The listing builds one solid part. Answer for the finished solid, in the listing's coordinates (mm). A direction names the side the tool comes from. Coordinates: 2 decimals unless noted, no trailing zeros. Loops run counter-clockwise (first coordinate to the right, second up) from the corner with the lowest first, then second, coordinate; pieces in that order, holes last. Notation, with made-up numbers: M -23.5,6 L 35.5,6 A20 cw 35.5,31 Z; hole C 33,-27.5 d6. An arc over 180 degrees is marked long. Answer in a Markdown table with one row per item. Add a question column.
from build123d import *

# Parameters (mm, degrees)
SKETCH1_R           = 5
BASEHEAD_DEPTH      = 6
SKETCH2_R           = 3
BASEBODY_DEPTH      = 20
HEXAGONSOCKET_DEPTH = 3
TOPFILLET_R         = 0.2
CHAMFER1_SIZE       = 0.1


with BuildPart() as part:
    # Sketch1 → BaseHead (new body)
    with BuildSketch(Plane(origin=(0, 0, 0), x_dir=(0, 0, -1), z_dir=(1, 0, 0))):
        Circle(SKETCH1_R)
    extrude(amount=BASEHEAD_DEPTH)

    # Sketch2 → BaseBody (add)
    with BuildSketch(Plane(origin=(6, 0, 0), x_dir=(0, 0, -1), z_dir=(1, 0, 0))):
        Circle(SKETCH2_R)
    extrude(amount=BASEBODY_DEPTH)

    # Sketch3 → HexagonSocket (cut)
    with BuildSketch(Plane(origin=(0, 0, 0), x_dir=(0, 0, -1), z_dir=(1, 0, 0))):
        Polygon((2.886751346, 0), (1.443375673, 2.5), (-1.443375673, 2.5), (-2.886751346, 0), (-1.443375673, -2.5), (1.443375673, -2.5), align=None)
    extrude(amount=HEXAGONSOCKET_DEPTH, mode=Mode.SUBTRACT)

    # Sketch4 → Cut-Revolve1 (revolve, cut)
    with BuildSketch(Plane(origin=(-4.19613823, 0.75, 0), x_dir=(-1, 0, 0), z_dir=(0, 0, 1))):
        Polygon((-7.19613823, 3.25), (-8.639513903, 0.75), (-7.19613823, 0.75), align=None)
    revolve(axis=Axis((0.838992387, 0, 0), (-1, 0, 0)), mode=Mode.SUBTRACT)

    # TopFillet
    topfillet_edges = [part.edges().sort_by_distance(p)[0] for p in [
        (0, 0, 5),
    ]]
    fillet(topfillet_edges, radius=TOPFILLET_R)

    # Chamfer1
    chamfer1_edges = [part.edges().sort_by_distance(p)[0] for p in [
        (26, 0, 3),
    ]]
    chamfer(chamfer1_edges, length=CHAMFER1_SIZE)


solid = part.part
(1) A cutting plane is placed at A-A (x = 2.25). Give the vertices of the cut face in (y, z).
(2) A cutting plane is placed at C-C (x = 5.5). Give the vertices of the cut face in (y, z), plus the area to 3 significant figures.
(3) For faces 1 (the face through (3.06, -4.88, 1.08)), 2 (the face through (6, -3.3, 0.1)), 3 (the face through (1.479, 1.233, -2.175)), determine the directions among +Z, -Z, +X, -X, +Y, -Y from which every point of the face is accessible in a straight line to the end or side of a thin tool.
(4) A cutting plane is placed at B-B (x = 18). Give the vertices of the cut face in (y, z), plus the area to 3 significant figures.
(5) Each of these flat-tipped pins is pushed along its axis until it touches: pin 1 (3 mm diameter, centred on x = 11, z = 4, fed in from +Y); pin 2 (6 mm diameter, centred on x = 12, y = -2.5, fed in from +Z); pin 3 (0.6 mm diameter, centred on y = 2, z = -1, fed in from -X). Where does it stop, or does it pass through?
(6) Straight lines are drawn through the part: line 1 (X direction, y = -4, z = 0.25); line 2 (Y direction, x = 3.25, z = 4); line 3 (Y direction, x = 7.25, z = -2). For each, find the intervals that lie inside material, in ascending order.
(7) The mould has two halves that part along Z. Classify faces 4 (the face through (16, 0, 3)), 5 (the face through (1.479, -1.267, -2.155)), 6 (the face through (1, -2.5, 0)), 7 (the face through (0, -2, -2)): released by +Z, released by -Z, zero draft, split by the parting line, or undercut.
Solved:
| question | item | result |
|---|---|---|
| 1 | outline | C 0,0 d10; hole M -2.5,-1.44 L 0,-2.89 L 2.5,-1.44 L 2.5,1.44 L 0,2.89 L -2.5,1.44 Z |
| 2 | outline | C 0,0 d10 |
| 2 | area | 78.5 mm² |
| 3 | face 1 | +X, -X |
| 3 | face 2 | +X |
| 3 | face 3 | -X |
| 4 | outline | C 0,0 d6 |
| 4 | area | 28.3 mm² |
| 5 | pin 1 | stops at y = 1.66 |
| 5 | pin 2 | stops at z = 3 |
| 5 | pin 3 | stops at x = 3 |
| 6 | line 1 | x = 0 to 6 |
| 6 | line 2 | y = -3 to 3 |
| 6 | line 3 | y = -2.24 to 2.24 |
| 7 | face 4 | split by the parting line |
| 7 | face 5 | undercut |
| 7 | face 6 | undercut |
| 7 | face 7 | zero draft |
